Autodesk Inventor part; units mm, degrees
ref_plane "Plano de trabalho1" through (0, 0, 0) normal (0, 0, 1) x (1, 0, 0)
ref_plane "YZ Plane" through (0, 0, 0) normal (1, 0, 0) x (0, 1, 0)
ref_plane "XZ Plane" through (0, 0, 0) normal (0, 1, 0) x (-1, 0, 0)
ref_plane "Plano de trabalho1" through (0, 0, 0) normal (0, 0, 1) x (1, 0, 0)
sketch "Esboço1" plane through (0, 0, 0) normal (0, 0, 1) x (1, 0, 0)
  arc A0 (-38.9725, -30.5146) -> (-28.9725, -40.5146) centre (-28.9725, -30.5146) ccw
  line L0 (31.0275, -40.5146) -> (-28.9725, -40.5146)
  arc A1 (31.0275, -40.5146) -> (41.0275, -30.5146) centre (31.0275, -30.5146) ccw
  line L1 (41.0275, 29.4854) -> (41.0275, -30.5146)
  arc A2 (41.0275, 29.4854) -> (31.0275, 39.4854) centre (31.0275, 29.4854) ccw
  line L2 (-28.9725, 39.4854) -> (31.0275, 39.4854)
  arc A3 (-28.9725, 39.4854) -> (-38.9725, 29.4854) centre (-28.9725, 29.4854) ccw
  line L3 (-38.9725, -30.5146) -> (-38.9725, 29.4854)
  circle A4 centre (1.0275, -0.5146) radius 5
  arc A5 (-52.2205, -30.5146) -> (-28.9725, -53.7625) centre (-28.9725, -30.5146) ccw
  line L4 (-52.2205, -30.5146) -> (-52.2205, 29.4854)
  arc A6 (-28.9725, 52.7334) -> (-52.2205, 29.4854) centre (-28.9725, 29.4854) ccw
  line L5 (-28.9725, 52.7334) -> (31.0275, 52.7334)
  arc A7 (54.2754, 29.4855) -> (31.0275, 52.7334) centre (31.0275, 29.4854) ccw
  line L6 (54.2754, 29.4855) -> (54.2754, -30.5145)
  arc A8 (31.0275, -53.7625) -> (54.2754, -30.5145) centre (31.0275, -30.5146) ccw
  line L7 (31.0275, -53.7625) -> (-28.9725, -53.7625)
  arc A9 (-59.6663, -30.5146) -> (-28.9725, -61.2084) centre (-28.9725, -30.5146) ccw
  line L8 (-59.6663, -30.5146) -> (-59.6664, 29.4854)
  arc A10 (-28.9725, 60.1793) -> (-59.6664, 29.4854) centre (-28.9725, 29.4854) ccw
  line L9 (-28.9725, 60.1793) -> (31.0275, 60.1793)
  arc A11 (61.7213, 29.4855) -> (31.0275, 60.1793) centre (31.0275, 29.4854) ccw
  line L10 (61.7213, 29.4855) -> (61.7213, -30.5145)
  arc A12 (31.0275, -61.2084) -> (61.7213, -30.5145) centre (31.0275, -30.5146) ccw
  line L11 (31.0275, -61.2084) -> (-28.9725, -61.2084)
  point P0 (0, 0)
extrude "Extrusão1" add sketch "Esboço1" along normal blind 30 contours L4 A6 L5 A7 L6 A8 L7 A5 | L8 A10 L9 A11 L10 A12 L11 A9
Can you work these out from the model? Positions are in its coordinate system, mm. A direction names the side the tool comes from. Give positions to 0.01 mm unless a question says otherwise; leave off trailing zeros. Order: outer loops, then holes, each group sorted by start corner. A loop starts at its lowest first (then second) coordinate and runs counter-clockwise, first axis right, second up. Notation, with made-up numbers: M -35.5,58 L -7.5,58 A27 cw -7.5,95 Z; hole C -27.5,84 d1. An arc over 180 degrees is marked long. Use a Markdown table: item, result. Add a question column.
Item 1: For faces 1 (the cylindrical face through (-35.97, -37.66, 14.79)), 2 (the cylindrical face through (52.49, 51.43, 14.79)), which set-ups out of +Z, -Z, +X, -X, +Y, -Y let a thin tool reach every point of the face, with its end or its side?
Item 2: Suppose I cut it at B-B (x = 1). List the corners of the cut face in (y, z) for me.
Item 3: If I drill on L1, parallel to Y at x = -16, z = 27.75; L2, parallel to X at y = -1, z = 4; L3, parallel to X at y = 32, z = 17.75, over which ranges is the centre line in solid material (lowest first)? Write a range as [from, to].
Item 4: Suppose I cut it at D-D (x = -46). List the corners of the cut face in (y, z) for me.
Item 5: Suppose I cut it at A-A (y = 27.5). List the corners of the cut face in (x, z) for me, then the cut area to 3 significant figures.
Item 6: Suppose I cut it at C-C (z = 24.5). List the corners of the cut face in (x, y) for me, then the cut area to 3 significant figures.
Item 7: We'd pull the mould along Y, two halves only. Please class faces 3 (the cylindrical face through (-50.914, 50.949, 14.79)), 4 (the flat face through (0, 41, 0)), 5 (the flat face through (1, 39.485, 15)): +Y half, -Y half, draft (parallel to the pull), parting line (faces both ways), or undercut.
Answer sheet:
| question | item | result |
|---|---|---|
| 1 | face 1 | +Z, -Z |
| 1 | face 2 | +Z, -Z, +X, +Y |
| 2 | outline | M -61.21,0 L -40.51,0 L -40.51,30 L -61.21,30 Z; M 39.49,0 L 60.18,0 L 60.18,30 L 39.49,30 Z |
| 3 | L1 | y = [-61.21, -40.51], [39.49, 60.18] |
| 3 | L2 | x = [-59.67, -38.97], [41.03, 61.72] |
| 3 | L3 | x = [-59.56, -38.65], [40.71, 61.62] |
| 4 | outline | M -56.05,0 L 55.02,0 L 55.02,30 L -56.05,30 Z |
| 5 | outline | M -59.67,0 L -38.97,0 L -38.97,30 L -59.67,30 Z; M 41.03,0 L 61.72,0 L 61.72,30 L 41.03,30 Z |
| 5 | area | 1,240 mm² |
| 6 | outline | M -59.67,-30.51 A30.69 ccw -28.97,-61.21 L 31.03,-61.21 A30.69 ccw 61.72,-30.51 L 61.72,29.49 A30.69 ccw 31.03,60.18 L -28.97,60.18 A30.69 ccw -59.67,29.49 Z; hole M -38.97,-30.51 A10 ccw -28.97,-40.51 L 31.03,-40.51 A10 ccw 41.03,-30.51 L 41.03,29.49 A10 ccw 31.03,39.49 L -28.97,39.49 A10 ccw -38.97,29.49 Z |
| 6 | area | 7,610 mm² |
| 7 | face 3 | +Y half |
| 7 | face 4 | draft |
| 7 | face 5 | undercut |
